Autodesk Inventor part; units mm, degrees
ref_plane "YZ Plane" through (0, 0, 0) normal (1, 0, 0) x (0, 1, 0)
ref_plane "XZ Plane" through (0, 0, 0) normal (0, 1, 0) x (-1, 0, 0)
ref_plane "XY Plane" through (0, 0, 0) normal (0, 0, 1) x (1, 0, 0)
sketch "Sketch1" plane through (0, 0, 0) normal (0, 0, 1) x (1, 0, 0)
  line L0 (20, -20) -> (20, 20) construction
  line L1 (20, 20) -> (-20, 20) construction
  line L2 (-20, 20) -> (-20, -20) construction
  line L3 (-20, -20) -> (20, 20) construction
  line L4 (20, -20) -> (-20, 20) construction
  line L5 (20, 20) -> (-20, 20)
  line L6 (20, 20) -> (20, -20)
  line L7 (-20, -20) -> (20, -20) construction
  line L8 (20, -20) -> (12, -20)
  line L9 (12, -20) -> (12, 12)
  line L10 (12, 12) -> (-20, 12)
  line L11 (-20, 20) -> (-20, 12)
  point P0 (0, 0)
  dimension "d0" = 40
  dimension "d1" = 40
  dimension "d3" = 8
extrude "Extrusion1" add sketch "Sketch1" along normal blind 41
sketch "Sketch2" plane through (0, 0, 41) normal (0, 0, 1) x (1, 0, 0)
  line L0 (20, 20) -> (-20, 20) construction
  line L1 (20, 20) -> (20, 16) construction
  line L2 (20, -20) -> (20, 20) construction
  line L3 (20, 16) -> (16, 16) construction
  line L4 (16, 16) -> (-8, 16) construction
  line L5 (16, 16) -> (16, -8) construction
  point P0 (0, 0)
  dimension "d6" = 4
  dimension "d7" = 4
  dimension "d8" = 24
  dimension "d9" = 24
hole "Hole1" at (-8, 16, 41) at (16, 16, 41) at (16, -8, 41) direction (0, 0, -1) diameter 4.3 depth 5 tip angle 118
properties part number "MirroHouseModel" material "Steel, Carbon"
Design review of the part built by this model. Coordinates are the model's own, in mm. A direction names the side the tool comes from. Coordinates: 2 decimals unless noted, no trailing zeros. Loops run counter-clockwise (first coordinate to the right, second up) from the corner with the lowest first, then second, coordinate; pieces in that order, holes last.
Item 1: Wall thickness on L1, parallel to X at y = 16, z = 39; L2, parallel to X at y = -8, z = 38: over which ranges is each line inside the solid? List them lowest first.
Completed:
L1: x = -20 to -10.15, -5.85 to 13.85, 18.15 to 20
L2: x = 12 to 13.85, 18.15 to 20
Item 2: Draft analysis for pull direction X (two halves, no side actions). For faces 4 (the flat face through (-20, 16, 20)), 5 (the flat face through (20, 0, 20)), 6 (the flat face through (16, -20, 20)), 7 (the cylindrical face through (18.1, 16.47, 38.47)), state which applies: pulls with the +X half, pulls with the -X half, needs draft (parallel to the pull), parting line crosses it, or undercut.
Completed:
face 4: pulls with the -X half
face 5: pulls with the +X half
face 6: needs draft
face 7: undercut
Item 3: Add section B-B (y = -15.5). Write out the cut boundary in (x, z), and give its area (3 significant figures).
Completed:
outline: (12, 0) - (20, 0) - (20, 41) - (12, 41) - close
area: 328 mm2
Item 4: Add section A-A (z = 5). Write out the cut boundary in (x, y), and give its area (3 significant figures).
Completed:
outline: (-20, 12) - (12, 12) - (12, -20) - (20, -20) - (20, 20) - (-20, 20) - close
area: 576 mm2
Item 5: Clearance check with flat-ended pins moving along their axes: pin 1 (5 mm diameter, centred on x = -12, z = 30, fed in from -Y); pin 2 (5 mm diameter, centred on y = 1.5, z = 14, fed in from -X). State where each tip first meets the part, or that it passes through.
Completed:
pin 1: stops at y = 12
pin 2: stops at x = 12
Item 6: For faces 1 (the flat face through (12, -4, 20)), 2 (the cylindrical face through (-9.81, 14.84, 38.47)), 3 (the flat face through (4, 14, 41)), list the 3-axis set-ups (+Z, -Z, +X, -X, +Y, -Y) from which the entire face can be reached by the end or side of a thin tool; tool diameter is ignored.
Completed:
face 1: +Z, -Z, -X, -Y
face 2: +Z
face 3: +Z, +X, -X, +Y, -Y
